```python
from build123d import *

# Parameters (mm, degrees)
SKETCH1_R           = 9
BOSS_EXTRUDE1_DEPTH = 4
SKETCH2_R           = 7
BOSS_EXTRUDE2_DEPTH = 3
BOSS_EXTRUDE2_TAPER = 30
CUT_EXTRUDE1_DEPTH  = 3
BOSS_EXTRUDE3_DEPTH = 40
SKETCH6_W           = 12
SKETCH6_H           = 23
CUT_EXTRUDE2_DEPTH  = 55.717456081
BOSS_EXTRUDE4_DEPTH = 3.5
SKETCH8_R           = 2
BOSS_EXTRUDE5_DEPTH = 3
SKETCH9_R           = 3.5
CUT_EXTRUDE3_DEPTH  = 52.720402164
BOSS_EXTRUDE6_DEPTH = 3.5
SKETCH11_R          = 2.45
BOSS_EXTRUDE7_DEPTH = 3.5
BOSS_EXTRUDE8_DEPTH = 3.5
FILLET3_START       = -26.84
FILLET3_DEPTH       = 2.84
FILLET3_START_2     = -12
FILLET3_2_DEPTH     = 2.83
FILLET3_START_3     = -21
FILLET3_3_DEPTH     = 21
FILLET3_START_4     = -27.84
FILLET3_4_DEPTH     = 1


with BuildPart() as part:
    # Sketch1 → Boss-Extrude1 (new body)
    with BuildSketch(Plane.XY):
        with BuildLine():
            Line((-35, -9), (0, -9))
            ThreePointArc((0, -9), (-8.437416666, -3.132091953), (-5.872614409, 6.82))
            ThreePointArc((-5.872614409, 6.82), (-19.465199243, -1.204217751), (-35, -4))
            Line((-35, -4), (-35, -9))
        make_face()
        Circle(SKETCH1_R)
    extrude(amount=BOSS_EXTRUDE1_DEPTH)

    # Sketch2 → Boss-Extrude2 (add)
    with BuildSketch(Plane(origin=(0, 0, 0), x_dir=(-1, 0, 0), z_dir=(0, 0, -1))):
        Circle(SKETCH2_R)
    extrude(amount=BOSS_EXTRUDE2_DEPTH, taper=BOSS_EXTRUDE2_TAPER)

    # Sketch4 → Cut-Extrude1 (cut)
    with BuildSketch(Plane.XY.offset(4)):
        with BuildLine():
            Line((1.2, -6.33), (1.8, -4.1378116))
            ThreePointArc((1.8, -4.1378116), (2.058560194, -3.569045514), (2.48, -3.1078116))
            ThreePointArc((2.48, -3.1078116), (2.64989874, -2.964295475), (2.811558399, -2.811558399))
            ThreePointArc((2.811558399, -2.811558399), (2.964295475, -2.64989874), (3.1078116, -2.48))
            ThreePointArc((3.1078116, -2.48), (3.569045514, -2.058560194), (4.1378116, -1.8))
            Line((4.1378116, -1.8), (6.33, -1.2))
            ThreePointArc((6.33, -1.2), (6.992020752, -0.754882576), (7.25, 0))
            ThreePointArc((7.25, 0), (6.992020752, 0.754882576), (6.33, 1.2))
            Line((6.33, 1.2), (4.1378116, 1.8))
            ThreePointArc((4.1378116, 1.8), (3.569045514, 2.058560194), (3.1078116, 2.48))
            ThreePointArc((3.1078116, 2.48), (2.964295475, 2.64989874), (2.811558399, 2.811558399))
            ThreePointArc((2.811558399, 2.811558399), (2.64989874, 2.964295475), (2.48, 3.1078116))
            ThreePointArc((2.48, 3.1078116), (2.058560194, 3.569045514), (1.8, 4.1378116))
            Line((1.8, 4.1378116), (1.2, 6.33))
            ThreePointArc((1.2, 6.33), (0.754882576, 6.992020752), (0, 7.25))
            ThreePointArc((0, 7.25), (-0.754882576, 6.992020752), (-1.2, 6.33))
            Line((-1.2, 6.33), (-1.8, 4.1378116))
            ThreePointArc((-1.8, 4.1378116), (-2.058560194, 3.569045514), (-2.48, 3.1078116))
            ThreePointArc((-2.48, 3.1078116), (-2.64989874, 2.964295475), (-2.811558399, 2.811558399))
            ThreePointArc((-2.811558399, 2.811558399), (-2.964295475, 2.64989874), (-3.1078116, 2.48))
            ThreePointArc((-3.1078116, 2.48), (-3.569045514, 2.058560194), (-4.1378116, 1.8))
            Line((-4.1378116, 1.8), (-6.33, 1.2))
            ThreePointArc((-6.33, 1.2), (-6.992020752, 0.754882576), (-7.25, 0))
            ThreePointArc((-7.25, 0), (-6.992020752, -0.754882576), (-6.33, -1.2))
            Line((-6.33, -1.2), (-4.1378116, -1.8))
            ThreePointArc((-4.1378116, -1.8), (-3.569045514, -2.058560194), (-3.1078116, -2.48))
            ThreePointArc((-3.1078116, -2.48), (-2.964295475, -2.64989874), (-2.811558399, -2.811558399))
            ThreePointArc((-2.811558399, -2.811558399), (-2.64989874, -2.964295475), (-2.48, -3.1078116))
            ThreePointArc((-2.48, -3.1078116), (-2.058560194, -3.569045514), (-1.8, -4.1378116))
            Line((-1.8, -4.1378116), (-1.2, -6.33))
            ThreePointArc((-1.2, -6.33), (-0.754882576, -6.992020752), (0, -7.25))
            ThreePointArc((0, -7.25), (0.754882576, -6.992020752), (1.2, -6.33))
        make_face()
    extrude(amount=-CUT_EXTRUDE1_DEPTH, mode=Mode.SUBTRACT)

    # Sketch5 → Boss-Extrude3 (add)
    with BuildSketch(Plane(origin=(0, 0, 0), x_dir=(-1, 0, 0), z_dir=(0, 0, -1))):
        with BuildLine():
            Line((35, -9), (35, -4))
            Line((35, -4), (9.17, -4))
            ThreePointArc((9.17, -4), (7.844486312, -6.205642902), (6, -8))
            Line((6, -8), (6, -9))
            Line((6, -9), (35, -9))
        make_face()
    extrude(amount=BOSS_EXTRUDE3_DEPTH)

    # Sketch6 → Cut-Extrude2 (cut, through all)
    with BuildSketch(Plane(origin=(0, -4, 0), x_dir=(1, 0, 0), z_dir=(0, 1, 0))):
        with Locations((-18, 20)):
            Rectangle(SKETCH6_W, SKETCH6_H)
    extrude(amount=-CUT_EXTRUDE2_DEPTH, mode=Mode.SUBTRACT)

    # Sketch7 → Boss-Extrude4 (add)
    with BuildSketch(Plane(origin=(0, -4, 0), x_dir=(1, 0, 0), z_dir=(0, 1, 0))):
        with BuildLine():
            Line((-28.5, 24), (-28.5, 16))
            ThreePointArc((-28.5, 16), (-31.5, 13), (-34.5, 16))
            Line((-34.5, 16), (-34.5, 24))
            ThreePointArc((-34.5, 24), (-31.5, 27), (-28.5, 24))
        make_face()
    extrude(amount=BOSS_EXTRUDE4_DEPTH)

    # Sketch8 → Boss-Extrude5 (add)
    with BuildSketch(Plane(origin=(0, -0.5, 0), x_dir=(1, 0, 0), z_dir=(0, 1, 0))):
        with Locations(Location((-31.5, 24, 0), (0, 0, 180))):
            Circle(SKETCH8_R)
        with Locations((-31.5, 16)):
            Circle(SKETCH8_R)
    extrude(amount=BOSS_EXTRUDE5_DEPTH)

    # Sketch9 → Cut-Extrude3 (cut, through all)
    with BuildSketch(Plane(origin=(0, 0, -3), x_dir=(-1, 0, 0), z_dir=(0, 0, -1))):
        Circle(SKETCH9_R)
    extrude(amount=-CUT_EXTRUDE3_DEPTH, mode=Mode.SUBTRACT)

    # Sketch10 → Boss-Extrude6 (add)
    with BuildSketch(Plane(origin=(0, -4, 0), x_dir=(1, 0, 0), z_dir=(0, 1, 0))):
        with BuildLine():
            Line((-26.84, 0), (-26.84, 20))
            Line((-26.84, 20), (-21.01, 20))
            ThreePointArc((-21.01, 20), (-18.010462475, 17.05267484), (-15.010924951, 20))
            Line((-15.010924951, 20), (-9.17, 20))
            Line((-9.17, 20), (-9.17, 0))
            Line((-9.17, 0), (-12, 0))
            Line((-12, 0), (-12, 3.75))
            ThreePointArc((-12, 3.75), (-11.25, 4.5), (-12, 5.25))
            Line((-12, 5.25), (-12, 11))
            Line((-12, 11), (-24, 11))
            Line((-24, 11), (-24, 5.25))
            ThreePointArc((-24, 5.25), (-24.75, 4.5), (-24, 3.75))
            Line((-24, 3.75), (-24, 0))
            Line((-24, 0), (-26.84, 0))
        make_face()
    extrude(amount=BOSS_EXTRUDE6_DEPTH)

    # Sketch11 → Boss-Extrude7 (add)
    with BuildSketch(Plane(origin=(0, -0.5, 0), x_dir=(1, 0, 0), z_dir=(0, 1, 0))):
        with Locations(Location((-18.006141049, 14.55267484, 0), (0, 0, 180))):
            Circle(SKETCH11_R)
    extrude(amount=BOSS_EXTRUDE7_DEPTH)

    # Sketch12 → Boss-Extrude8 (add)
    with BuildSketch(Plane(origin=(0, -4, 0), x_dir=(1, 0, 0), z_dir=(0, 1, 0))):
        Polygon((-20.68, 4.2), (-23.5, 4.2), (-21.5, 7), (-18.05, 3.55), (-17.95, 3.55), (-14.5, 7), (-12.5, 4.2), (-15.32, 4.2), (-16.25, 1), (-17.97, 3.45), (-18.03, 3.45), (-19.75, 1), align=None)
    extrude(amount=BOSS_EXTRUDE8_DEPTH)

    # Fillet3: read off the stored shape, not the designer's step
    # Fillet3 outline → Fillet3 (add)
    with BuildSketch(Plane.YZ.offset(FILLET3_START)):
        with BuildLine():
            ThreePointArc((-4, -21), (-3.707106781, -20.292893219), (-3, -20))
            Line((-3, -20), (-4, -20))
            Line((-4, -20), (-4, -21))
        make_face()
    extrude(amount=FILLET3_DEPTH)

    # Fillet3 2 outline → Fillet3 2 (add)
    with BuildSketch(Plane.YZ.offset(FILLET3_START_2)):
        with BuildLine():
            ThreePointArc((-4, -21), (-3.707106781, -20.292893219), (-3, -20))
            Line((-3, -20), (-4, -20))
            Line((-4, -20), (-4, -21))
        make_face()
    extrude(amount=FILLET3_2_DEPTH)

    # Fillet3 3 outline → Fillet3 3 (add)
    with BuildSketch(Plane.XY.offset(FILLET3_START_3)):
        with BuildLine():
            Line((-26.84, -4), (-26.84, -3))
            ThreePointArc((-26.84, -3), (-27.132893219, -3.707106781), (-27.84, -4))
            Line((-27.84, -4), (-26.84, -4))
        make_face()
    extrude(amount=FILLET3_3_DEPTH)

    # Fillet3 4 outline → Fillet3 4 (cut)
    with BuildSketch(Plane.YZ.offset(FILLET3_START_4)):
        with BuildLine():
            Line((-2, -19.999999999), (-3, -20))
            ThreePointArc((-3, -20), (-3.707106781, -20.292893219), (-4, -21))
            Line((-4, -21), (-2, -21))
            Line((-2, -21), (-2, -19.999999999))
        make_face()
    extrude(amount=FILLET3_4_DEPTH, mode=Mode.SUBTRACT)


solid = part.part
```
Check sheet for the modelled part. Datum: model origin and axes. Units: mm. A direction names the side the tool comes from. Give positions to 0.01 mm unless a question says otherwise; leave off trailing zeros. Order: outer loops, then holes, each group sorted by start corner. A loop starts at its lowest first (then second) coordinate and runs counter-clockwise, first axis right, second up. Notation, with made-up numbers: (-28.75, -33.75) -> (19.25, -33.75) arc R19 cw to (19.25, -26.75) -> close; hole circle Ø9 at (13, 83.5). An arc over 180 degrees is marked (long way). Return JSON: item names as keys, results as strings.
1. Cross-section at C-C, the plane x = -26. Record the cut outline in (y, z).
From the geometry:
{"outline": "(-9, -40) -> (-4, -40) -> (-4, -21) arc R1 cw to (-3, -20) -> (-0.5, -20) -> (-0.5, 0) -> (-3.08, 0) -> (-3.08, 4) -> (-9, 4) -> close"}
2. Set-up check for faces 1 (the flat face through (-24, -2, -20)), 2 (the cylindrical face through (-33.408, 0.979, -23.399)), 3 (the cylindrical face through (0.746, -6.999, 2.521)), 4 (the flat face through (-31, 2.5, -24)): record each of +Z, -Z, +X, -X, +Y, -Y from which the full face is reachable in a straight line by a thin tool's end or side.
From the geometry:
{"face 1": "-Z, +Y", "face 2": "+Y", "face 3": "+Z", "face 4": "+Z, -Z, +X, -X, +Y"}
3. Mould release check, pull along Z, two halves, no side actions. Record for faces 5 (the cylindrical face through (-18.076, -2.274, -17.053)), 6 (the flat face through (-18, -6, -31.5)), 7 (the flat face through (-5.249, -1.496, 2.521)): +Z half, -Z half, draft (parallel to the pull), parting line (faces both ways), or undercut.
From the geometry:
{"face 5": "-Z half", "face 6": "undercut", "face 7": "draft"}
4. Cross-section at B-B, the plane z = -33. Record the cut outline in (x, y), plus the area to 3 significant figures.
From the geometry:
{"outline": "(-35, -9) -> (-6, -9) -> (-6, -8) arc R10 cw to (-9.17, -4) -> (-35, -4) -> close", "area": "138 mm^2"}
5. Cross-section at A-A, the plane z = -28.5. Record the cut outline in (x, y), plus the area to 3 significant figures.
From the geometry:
{"outline": "(-35, -9) -> (-24, -9) -> (-24, -4) -> (-35, -4) -> close; (-12, -9) -> (-6, -9) -> (-6, -8) arc R10 cw to (-9.17, -4) -> (-12, -4) -> close", "area": "77.5 mm^2"}
6. Material ranges on probe 1 along Z at (x, y) = (-19.5, -7); probe 2 along Z at (x, y) = (-2, 8); probe 3 along X at (y, z) = (-2.75, -14.5), recorded low to high. Write a range as [from, to].
From the geometry:
{"probe 1": "[-40, -31.5], [-8.5, 4]", "probe 2": "[0, 4]", "probe 3": "[-34.1, -28.9], [-26.84, -9.17]"}
7. Go/stop test with flat-tipped pins: P1, Ø3, axis at y = -2, z = -19.5, coming from the +X side; P2, Ø10, axis at x = -19, z = -20.5, coming from the +Y side; P3, Ø2, axis at x = -31, z = -23, coming from the +Y side; P4, Ø7, axis at y = -3, z = -22.5, coming from the -X side. Record where each tip stops, or that it passes through.
From the geometry:
{"P1": "x = -9.17", "P2": "y = 3", "P3": "y = 2.5", "P4": "x = -35"}
8. Cross-section at D-D, the plane x = -31.5. Record the cut outline in (y, z), plus the area to 3 significant figures.
From the geometry:
{"outline": "(-9, -40) -> (-4, -40) -> (-4, -27) -> (-0.5, -27) -> (-0.5, -26) -> (2.5, -26) -> (2.5, -22) -> (-0.5, -22) -> (-0.5, -18) -> (2.5, -18) -> (2.5, -14) -> (-0.5, -14) -> (-0.5, -13) -> (-4, -13) -> (-4, 0) -> (-3.86, 0) -> (-3.86, 4) -> (-9, 4) -> close", "area": "294 mm^2"}
